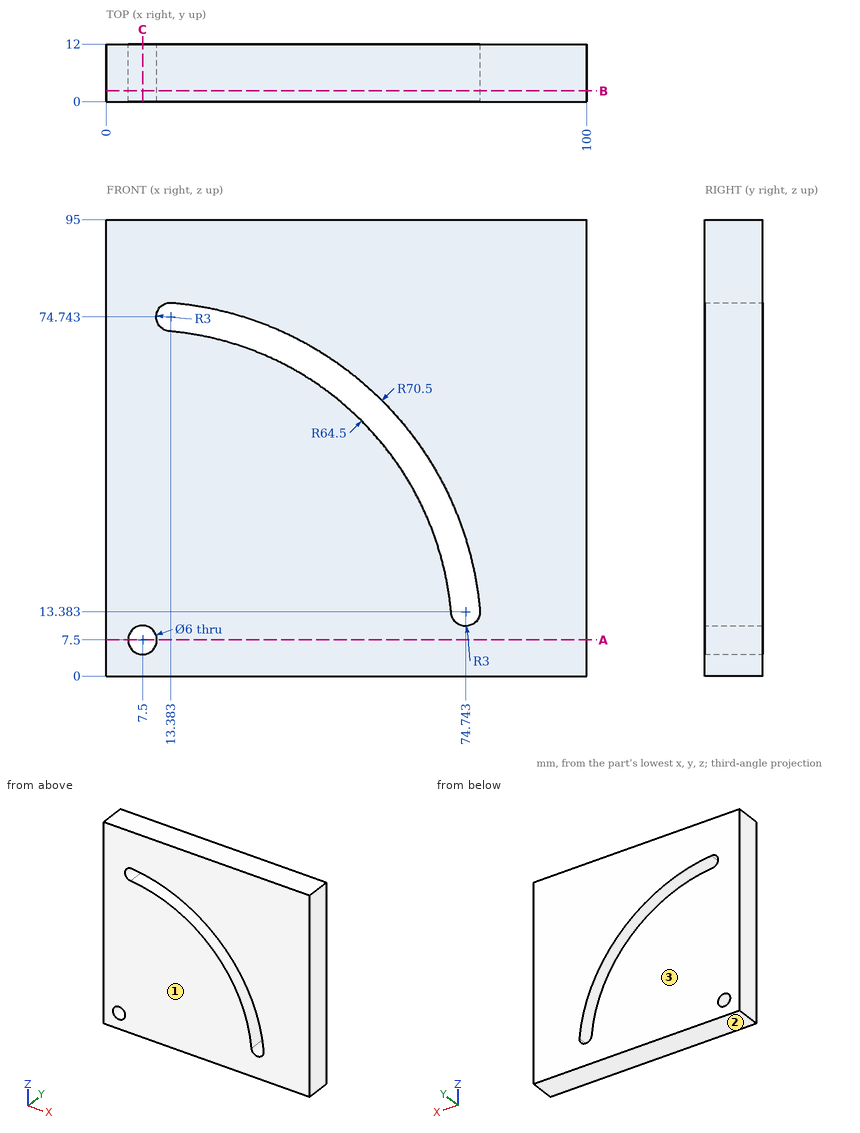
Print and shaded views of the part. All mm, measured from the part's lowest x, y and z. Coordinates: 2 decimals unless noted, no trailing zeros. Loops run counter-clockwise (first coordinate to the right, second up) from the corner with the lowest first, then second, coordinate; pieces in that order, holes last. Notation, with made-up numbers: M 71,-1 L 108,-1 A29 ccw 108,35 Z; hole C 82,-29.75 d5. An arc over 180 degrees is marked long. Use a Markdown table: item, result. Add a question column.
Q1. Mould opens along Y. For the marked faces 1, 2 and 3 say: +Y half, -Y half, draft (parallel to the pull), parting line (faces both ways), or undercut.
Q2. Cut at C-C (x = 7.5). Write the cut outline in (y, z).
Q3. Cut at B-B (y = 2.25). Write the cut outline in (x, z), and give its area (3 significant figures).
Q4. Cut at A-A (z = 7.5). Write the cut outline in (x, y), and give its area (3 significant figures).
Q5. Probe L1, parallel to Z at x = 7.5, y = 2.75; L2, parallel to X at y = 11.25, z = 56.5; L3, parallel to Z at x = 64, y = 1.5 (1 decimal). List the from-to ranges inside material, lowest first.
Worked out:
| question | item | result |
|---|---|---|
| 1 | face 1 | -Y half |
| 1 | face 2 | draft |
| 1 | face 3 | +Y half |
| 2 | outline | M 0,0 L 12,0 L 12,4.5 L 0,4.5 Z; M 0,10.5 L 12,10.5 L 12,95 L 0,95 Z |
| 3 | outline | M 0,0 L 100,0 L 100,95 L 0,95 Z; hole C 7.5,7.5 d6; hole M 13.12,71.75 A64.5 cw 71.75,13.12 A3 ccw 77.73,13.64 A70.5 ccw 13.64,77.73 A3 ccw Z |
| 3 | area | 8,880 mm2 |
| 4 | outline | M 0,0 L 4.5,0 L 4.5,12 L 0,12 Z; M 10.5,0 L 100,0 L 100,12 L 10.5,12 Z |
| 4 | area | 1,130 mm2 |
| 5 | L1 | z = 0 to 4.5, 10.5 to 95 |
| 5 | L2 | x = 0 to 49.44, 58.19 to 100 |
| 5 | L3 | z = 0 to 38.6, 49.7 to 95 |
